Source: CAD feature listing. Evaluate the final solid. Frame: model axes, mm. A direction names the side the tool comes from. Give positions to 0.01 mm unless a question says otherwise; leave off trailing zeros. Write each loop counter-clockwise with the first axis right and the second up, starting at its lowest first coordinate (ties: lowest second). Pieces come first, ordered by that corner, then holes. Notation, with made-up numbers: (32.5, 23) -> (56.5, 23) arc R16 ccw to (56.5, 29) -> close; hole circle Ø10 at (-31.75, -37.75). An arc over 180 degrees is marked (long way). Write item = value, one per line.
from build123d import *

# Parameters (mm, degrees)
SKETCH_W        = 18
SKETCH_H        = 20
PAD_DEPTH       = 4.5
SKETCH001_W     = 9
SKETCH001_H     = 5
PAD001_DEPTH    = 23
SKETCH002_W     = 9
SKETCH002_H     = 6
PAD002_DEPTH    = 23
SKETCH004_W     = 2
SKETCH004_H     = 6
SKETCH004_H_2   = 5
PAD003_DEPTH    = 12
SKETCH005_R     = 1.3
POCKET_DEPTH    = 25
SKETCH007_W     = 2
SKETCH007_H     = 12
PAD004_DEPTH    = 7.2
SKETCH008_R     = 1.3
POCKET001_DEPTH = 5
COPYSKETCH009_R = 1.7
POCKET002_DEPTH = 5
SKETCH010_R     = 2.7
POCKET003_DEPTH = 2.7
SKETCH011_R     = 1.7
POCKET004_DEPTH = 7


with BuildPart() as part:
    # Sketch → Pad (new body)
    with BuildSketch(Plane.XY):
        Rectangle(SKETCH_W, SKETCH_H)
    extrude(amount=PAD_DEPTH)

    # Sketch001 (on Face6 of Pad) → Pad001 (join)
    with BuildSketch(Plane.XY.offset(4.5)):
        with Locations((4.5, -5.7)):
            Rectangle(SKETCH001_W, SKETCH001_H)
    extrude(amount=PAD001_DEPTH)

    # Sketch002 (on Face5 of Pad001) → Pad002 (join)
    with BuildSketch(Plane.XY.offset(4.5)):
        with Locations((4.5, 7)):
            Rectangle(SKETCH002_W, SKETCH002_H)
    extrude(amount=PAD002_DEPTH)

    # Sketch004 (on Face15 of Pad002) → Pad003 (join)
    with BuildSketch(Plane.XY.offset(27.5)):
        with Locations((8, 7)):
            Rectangle(SKETCH004_W, SKETCH004_H)
        with Locations((8, -5.7)):
            Rectangle(SKETCH004_W, SKETCH004_H_2)
    extrude(amount=PAD003_DEPTH)

    # Sketch005 (on Face10 of Pad003) → Pocket (cut)
    with BuildSketch(Plane.XZ.offset(8.2)):
        with Locations((4.5, 18.9)):
            Circle(SKETCH005_R)
        with Locations((4.5, 9.5)):
            Circle(SKETCH005_R)
    extrude(amount=-POCKET_DEPTH, mode=Mode.SUBTRACT)

    # Sketch007 → Pad004 (join)
    with BuildSketch(Plane.XZ.offset(-4)):
        with Locations((8, 33.5)):
            Rectangle(SKETCH007_W, SKETCH007_H)
    extrude(amount=PAD004_DEPTH)

    # Sketch008 (on Face31 of Pad004) → Pocket001 (cut)
    with BuildSketch(Plane(origin=(7, 0, 0), x_dir=(0, -1, 0), z_dir=(-1, 0, 0))):
        with Locations((-4.782348, 35.5)):
            Circle(SKETCH008_R)
        with Locations((4.617652, 35.5)):
            Circle(SKETCH008_R)
    extrude(amount=-POCKET001_DEPTH, mode=Mode.SUBTRACT)

    # CopySketch009 → Pocket002 (cut)
    with BuildSketch(Plane.XY.offset(4.5)):
        with Locations((-5.02174, 0)):
            Circle(COPYSKETCH009_R)
    extrude(amount=-POCKET002_DEPTH, mode=Mode.SUBTRACT)

    # Sketch010 (on Face5 of Pocket002) → Pocket003 (cut)
    with BuildSketch(Plane.XY.offset(4.5)):
        with Locations((-5.02174, 0)):
            Circle(SKETCH010_R)
    extrude(amount=-POCKET003_DEPTH, mode=Mode.SUBTRACT)

    # Sketch011 (on Face6 of Pocket003) → Pocket004 (cut)
    with BuildSketch(Plane(origin=(0, 10, 0), x_dir=(-1, 0, 0), z_dir=(0, 1, 0))):
        with Locations((-4.5, 18.9)):
            Circle(SKETCH011_R)
        with Locations((-4.5, 9.5)):
            Circle(SKETCH011_R)
    extrude(amount=-POCKET004_DEPTH, mode=Mode.SUBTRACT)


solid = part.part
(1) First-contact query: pin 1 (3.5 mm diameter, centred on y = -2, z = 31, fed in from -X); pin 2 (1.8 mm diameter, centred on x = 5, y = 7.5, fed in from +Z); pin 3 (6.5 mm diameter, centred on y = 8.5, z = 18.5, fed in from -X); pin 4 (2 mm diameter, centred on y = 4.78, z = 35.5, fed in from +X). Flat tips, straight axial feed; report the tip coordinate or a pass-through.
Values follow:
pin_1 = 7
pin_2 = 27.5
pin_3 = 0
pin_4 = through
(2) Pull-direction query (Z, two-part tool) for faces 4 (the face through (0, 0, 0)), 5 (the face through (7.986, 4.083, 36.596)), 6 (the face through (3, -8.2, 18)); classes: pulls with the +Z half, pulls with the -Z half, needs draft (parallel to the pull), parting line crosses it, or undercut.
Values follow:
face_4 = pulls with the -Z half
face_5 = undercut
face_6 = needs draft
(3) Section query B-B (z = 35.5). Return loops of the section in (x, y), plus the area to 3 significant figures.
Values follow:
outline = (7, -8.2) -> (9, -8.2) -> (9, -5.92) -> (7, -5.92) -> close; (7, -3.32) -> (9, -3.32) -> (9, 3.48) -> (7, 3.48) -> close; (7, 6.08) -> (9, 6.08) -> (9, 10) -> (7, 10) -> close
area = 26.0 mm2
(4) Section query D-D (z = 24). Return loops of the section in (x, y).
Values follow:
outline = (0, -8.2) -> (9, -8.2) -> (9, -3.2) -> (0, -3.2) -> close; (0, 4) -> (9, 4) -> (9, 10) -> (0, 10) -> close
(5) Section query A-A (x = 4.5). Return loops of the section in (y, z).
Values follow:
outline = (-10, 0) -> (10, 0) -> (10, 7.8) -> (4, 7.8) -> (4, 4.5) -> (-3.2, 4.5) -> (-3.2, 8.2) -> (-8.2, 8.2) -> (-8.2, 4.5) -> (-10, 4.5) -> close; (-8.2, 10.8) -> (-3.2, 10.8) -> (-3.2, 17.6) -> (-8.2, 17.6) -> close; (-8.2, 20.2) -> (-3.2, 20.2) -> (-3.2, 27.5) -> (-8.2, 27.5) -> close; (4, 11.2) -> (10, 11.2) -> (10, 17.2) -> (4, 17.2) -> close; (4, 20.6) -> (10, 20.6) -> (10, 27.5) -> (4, 27.5) -> close
(6) Access query for faces 1 (the face through (4.87, 7.04, 17.24)), 2 (the face through (3, -6, 27.5)), 3 (the face through (-3, 0, 1.8)). Directions: +Z, -Z, +X, -X, +Y, -Y. A direction counts if a zero-diameter tool reaches every point of the face in a straight line with its end or side. Return the directions, or none.
Values follow:
face_1 = +Y
face_2 = +Z, -X, +Y, -Y
face_3 = +Z
(7) Material intervals for line 1 (Z direction, x = 4.5, y = -5.05); line 2 (Z direction, x = 4.5, y = 6.85); line 3 (Y direction, x = 7.25, z = 36), sorted ascending.
Values follow:
line_1 = 0 to 8.2, 10.8 to 17.6, 20.2 to 27.5
line_2 = 0 to 7.8, 11.2 to 17.2, 20.6 to 27.5
line_3 = -8.2 to -5.82, -3.42 to 3.58, 5.98 to 10
(8) Section query C-C (y = 5). Return loops of the section in (x, z).
Values follow:
outline = (-9, 0) -> (9, 0) -> (9, 34.22) -> (7, 34.22) -> (7, 27.5) -> (0, 27.5) -> (0, 4.5) -> (-9, 4.5) -> close; (7, 36.78) -> (9, 36.78) -> (9, 39.5) -> (7, 39.5) -> close; hole circle Ø3.4 at (4.5, 9.5); hole circle Ø3.4 at (4.5, 18.9)
